Geometry: final body of the model. Coordinates: model frame, mm. A direction names the side the tool comes from. Give positions to 0.01 mm unless a question says otherwise; leave off trailing zeros. Loops run counter-clockwise (first coordinate to the right, second up) from the corner with the lowest first, then second, coordinate; pieces in that order, holes last. Notation, with made-up numbers: M 74.5,43 L 85.5,43 A12 ccw 85.5,50 Z; hole C 47.5,41.5 d9. An arc over 180 degrees is marked long. Put each result on its own line as item: value.
```python
from build123d import *

# Parameters (mm, degrees)
SKETCH1_R           = 1.1
BOSS_EXTRUDE1_DEPTH = 0.8
FILLET1_R           = 1


with BuildPart() as part:
    # Sketch1 → Boss-Extrude1 (new, symmetric)
    with BuildSketch(Plane.XY):
        with BuildLine():
            Line((0.75, 1.418659837), (14.721500475, -0.364074443))
            ThreePointArc((14.721500475, -0.364074443), (16.234415683, -2.333028406), (14.255453949, -3.832829256))
            Line((14.255453949, -3.832829256), (12.712907233, -3.615136886))
            Line((12.712907233, -3.615136886), (10.312842352, -3.276427006))
            ThreePointArc((10.312842352, -3.276427006), (9.698394701, -2.942897128), (9.452585289, -2.288400506))
            add(Edge.make_bspline(
                [(9.452585289, -2.288400506), (9.450870019, -1.494900378), (8.489042718, 0.058923345), (4.930908227, -2.300819074), (2.487654104, -2.172094957), (1.138622907, -1.981712523)],
                knots=[0.051353436, 0.051353436, 0.051353436, 0.051353436, 0.215328782, 0.591995085, 1, 1, 1, 1], degree=3))
            Line((1.138622907, -1.981712523), (-1.75, -1.574054745))
            Line((-1.75, -1.574054745), (-1.75, 4.925945255))
            Line((-1.75, 4.925945255), (0.75, 4.925945255))
            Line((0.75, 4.925945255), (0.75, 1.418659837))
        make_face()
        with Locations((14.5, -2.1)):
            Circle(SKETCH1_R, mode=Mode.SUBTRACT)
        Circle(SKETCH1_R, mode=Mode.SUBTRACT)
    extrude(amount=BOSS_EXTRUDE1_DEPTH, both=True)

    # Fillet1
    fillet1_edges = [part.edges().sort_by_distance(p)[0] for p in [
        (0.75, 1.418659837, 0),
        (-1.75, -1.574054745, 0),
        (-1.75, 4.925945255, 0),
        (0.75, 4.925945255, 0),
    ]]
    fillet(fillet1_edges, radius=FILLET1_R)


solid = part.part
```
Item 1: Section A-A on x = 14.5. Output: boundary loops of the cut face in (y, z).
Output values:
outline: M -3.85,-0.8 L -3.2,-0.8 L -3.2,0.8 L -3.85,0.8 Z; M -1,-0.8 L -0.34,-0.8 L -0.34,0.8 L -1,0.8 Z
Item 2: Section D-D on y = 1.5. Output: boundary loops of the cut face in (x, z), then the cut area to 3 significant figures.
Output values:
outline: M -1.75,-0.8 L 1.15,-0.8 L 1.15,0.8 L -1.75,0.8 Z
area: 4.64 mm²
Item 3: Section B-B on y = 0. Output: boundary loops of the cut face in (x, z).
Output values:
outline: M -1.75,-0.8 L -1.1,-0.8 L -1.1,0.8 L -1.75,0.8 Z; M 1.1,-0.8 L 11.87,-0.8 L 11.87,0.8 L 1.1,0.8 Z
Item 4: Pin query (flat end, axial travel): pin 1 Ø2 at (x, y) = (14, -2.5) entering from +Z; pin 2 Ø0.8 at (y, z) = (3, 0) entering from +X. Return the tip coordinate at first contact, or that it passes through.
Output values:
pin 1: z = 0.8
pin 2: x = 0.75
Item 5: Mould query, pull axis Y, two halves, no side actions, for faces 1 (the cylindrical face through (13.4, -2.1, 0)), 2 (the flat face through (-1.75, 2, 0)), 3 (the flat face through (8.081, 0.483, 0.011)), 4 (the cylindrical face through (-1.498, -1.369, 0.011)). Classes: pulls with the +Y half, pulls with the -Y half, needs draft (parallel to the pull), parting line crosses it, or undercut.
Output values:
face 1: undercut
face 2: needs draft
face 3: pulls with the +Y half
face 4: pulls with the -Y half
Item 6: Section C-C on z = -0.6. Count the separate pieces of the cut face and the enclosed holes in it, then the cut area to 3 significant figures.
Output values:
separate pieces: 1
enclosed holes: 2
area: 52.1 mm²
Item 7: Set-up query: faces 5 (the flat face through (0.14, -1.84, 0.01)), 6 (the flat face through (0.75, 3, 0)). Return all of +Z, -Z, +X, -X, +Y, -Y with unobstructed straight access to the full face (end or side cutting, diameter ignored); none if empty.
Output values:
face 5: +Z, -Z, -X, -Y
face 6: +Z, -Z, +X, +Y
Item 8: Line query: probe 1 along X at (y, z) = (2.5, 0.05); probe 2 along X at (y, z) = (-2.5, 0.1); probe 3 along Y at (x, z) = (0, 0.55). Output: solid intervals per line, ascending. Write a range as [from, to].
Output values:
probe 1: [-1.75, 0.75]
probe 2: [9.48, 13.48], [15.52, 16.2]
probe 3: [-1.82, -1.1], [1.1, 4.89]
